The listing builds one solid part. Answer for the finished solid, in the listing's coordinates (mm). A direction names the side the tool comes from. Give positions to 0.01 mm unless a question says otherwise; leave off trailing zeros. Loops run counter-clockwise (first coordinate to the right, second up) from the corner with the lowest first, then second, coordinate; pieces in that order, holes last. Notation, with made-up numbers: M 86.25,72.5 L 127.25,72.5 A9 cw 127.25,82.5 Z; hole C 60,22.25 d7. An arc over 180 degrees is marked long. Use one line per item in the form item = value. Start each with the question number.
1. The part is cut by section D-D (x = 43). Write down the section's boundary in (y, z), and give its area (3 significant figures).
2. The part is cut by section A-A (z = 66.5). Write down the section's boundary in (x, y), and give its area (3 significant figures).
3. The part is cut by section C-C (z = 20). Give the number of separate pieces and of enclosed holes in the cut face, and give its area (3 significant figures).
4. Straight lines are drawn through the part: line 1 (X direction, y = -25.5, z = 46); line 2 (X direction, y = -80.5, z = 25); line 3 (Z direction, x = -117, y = 64). For each, find the intervals that lie inside material, in ascending order. Write a range as from..to.
5. The mould has two halves that part along X. Classify faces 5 (the face through (-118, -107.883, 26)), 6 (the face through (141.234, 24, 40)), 7 (the face through (125, -107.883, 26)), 8 (the face through (130, -24.883, 30)): released by +X, released by -X, zero draft, split by the parting line, or undercut.
6. For faces 1 (the face through (127, -19.883, 27)), 2 (the face through (-118, 65.117, 26)), 3 (the face through (-133.766, 24, 40)), 4 (the face through (24.2, -112.883, 4.5)), determine the directions among +Z, -Z, +X, -X, +Y, -Y from which every point of the face is accessible in a straight line to the end or side of a thin tool.
7. The part is cut by section B-B (y = 20). Write down the section's boundary in (x, z).
8. Each of these flat-tipped pins is pushed along its axis until it touches: pin 1 Ø1 at (y, z) = (-47, 14) entering from -X; pin 2 Ø24 at (y, z) = (-57, 29) entering from +X; pin 3 Ø13.5 at (x, z) = (128, 40.5) entering from +Y. Where does it stop, or does it pass through?
from build123d import *

# Parameters (mm, degrees)
SKETCH1_W                = 285
SKETCH1_H                = 188
BOSS_EXTRUDE1_DEPTH      = 5
SKETCH3_W                = 5
SKETCH3_H                = 90
BOSS_EXTRUDE2_DEPTH      = 72
SKETCH6_W                = 40
SKETCH6_H                = 5
BOSS_EXTRUDE3_DEPTH      = 10
SKETCH7_W                = 12
SKETCH7_H                = 5
BOSS_EXTRUDE4_DEPTH      = 45
SKETCH8_W                = 40
SKETCH8_H                = 5
BOSS_EXTRUDE5_DEPTH      = 72
CUT_EXTRUDE4_DEPTH       = 94
CUT_EXTRUDE4_DEPTH_BACK  = 96
SKETCH13_W               = 5
SKETCH13_H               = 90
BOSS_EXTRUDE6_DEPTH      = 72
SKETCH14_W               = 40
SKETCH14_H               = 5
BOSS_EXTRUDE7_DEPTH      = 55
SKETCH16_W               = 28
SKETCH16_H               = 45
CUT_EXTRUDE5_DEPTH       = 179
CUT_EXTRUDE5_DEPTH_BACK  = 11
SKETCH17_W               = 40
SKETCH17_H               = 5
BOSS_EXTRUDE9_DEPTH      = 55
SKETCH21_W               = 27.761976985
SKETCH21_H               = 40
CUT_EXTRUDE6_DEPTH       = 91
CUT_EXTRUDE6_DEPTH_BACK  = 99
SKETCH22_W               = 5
SKETCH22_H               = 88
BOSS_EXTRUDE10_DEPTH     = 80
SKETCH23_W               = 40
SKETCH23_H               = 5
BOSS_EXTRUDE11_DEPTH     = 55
SKETCH25_W               = 27.891782469
SKETCH25_H               = 44.37316573
CUT_EXTRUDE7_DEPTH       = 184
CUT_EXTRUDE7_DEPTH_BACK  = 6
SKETCH26_W               = 40
SKETCH26_H               = 5
BOSS_EXTRUDE12_DEPTH     = 55
SKETCH27_W               = 28
SKETCH27_H               = 45
CUT_EXTRUDE9_DEPTH       = 101
CUT_EXTRUDE9_DEPTH_BACK  = 89
SKETCH29_W               = 5
SKETCH29_H               = 88
BOSS_EXTRUDE14_DEPTH     = 80
SKETCH30_W               = 40
SKETCH30_H               = 5
BOSS_EXTRUDE15_DEPTH     = 55
SKETCH31_W               = 27.846515173
SKETCH31_H               = 45
CUT_EXTRUDE10_DEPTH      = 184
CUT_EXTRUDE10_DEPTH_BACK = 6
SKETCH32_W               = 40
SKETCH32_H               = 5
BOSS_EXTRUDE16_DEPTH     = 55
SKETCH33_W               = 27.846515173
SKETCH33_H               = 45
CUT_EXTRUDE11_DEPTH      = 84
CUT_EXTRUDE11_DEPTH_BACK = 106
SKETCH36_W               = 15
SKETCH36_H               = 5
CUT_EXTRUDE12_DEPTH      = 1
CUT_EXTRUDE12_DEPTH_BACK = 7


with BuildPart() as part:
    # Sketch1 → Boss-Extrude1 (new body)
    with BuildSketch(Plane.XY):
        with Locations((3.734064661, -18.883040936)):
            Rectangle(SKETCH1_W, SKETCH1_H)
    extrude(amount=BOSS_EXTRUDE1_DEPTH)

    # Sketch3 → Boss-Extrude2 (add)
    with BuildSketch(Plane.XY.offset(5)):
        with Locations((-131.265935339, 25.116959064)):
            Rectangle(SKETCH3_W, SKETCH3_H)
    extrude(amount=BOSS_EXTRUDE2_DEPTH)

    # Sketch6 → Boss-Extrude3 (add)
    with BuildSketch(Plane.XY.offset(5)):
        with Locations((-108.765935339, 67.616959064)):
            Rectangle(SKETCH6_W, SKETCH6_H)
    extrude(amount=BOSS_EXTRUDE3_DEPTH)

    # Sketch7 → Boss-Extrude4 (add)
    with BuildSketch(Plane.XY.offset(15)):
        with Locations((-122.765935339, 67.616959064)):
            Rectangle(SKETCH7_W, SKETCH7_H)
    extrude(amount=BOSS_EXTRUDE4_DEPTH)

    # Sketch8 → Boss-Extrude5 (add)
    with BuildSketch(Plane.XY.offset(77)):
        with Locations((-108.765935339, -17.383040936)):
            Rectangle(SKETCH8_W, SKETCH8_H)
    extrude(amount=-BOSS_EXTRUDE5_DEPTH)

    # Sketch9 → Cut-Extrude4 (cut, two sides)
    with BuildSketch(Plane.XZ.offset(19.883040936)) as cut_extrude4_sk:
        Polygon((-116.765935339, 15), (-88.765935339, 15), (-88.765935339, 77), (-128.765935339, 77), (-128.765935339, 60), (-116.765935339, 60), align=None)
    extrude(amount=CUT_EXTRUDE4_DEPTH, mode=Mode.SUBTRACT)
    extrude(cut_extrude4_sk.sketch, amount=-CUT_EXTRUDE4_DEPTH_BACK, mode=Mode.SUBTRACT)

    # Sketch13 → Boss-Extrude6 (add)
    with BuildSketch(Plane.XY.offset(5)):
        with Locations((138.734064661, 25.116959064)):
            Rectangle(SKETCH13_W, SKETCH13_H)
    extrude(amount=BOSS_EXTRUDE6_DEPTH)

    # Sketch14 → Boss-Extrude7 (add)
    with BuildSketch(Plane.XY.offset(5)):
        with Locations((116.234064661, 67.616959064)):
            Rectangle(SKETCH14_W, SKETCH14_H)
    extrude(amount=BOSS_EXTRUDE7_DEPTH)

    # Sketch16 → Cut-Extrude5 (cut, two sides)
    with BuildSketch(Plane.XZ.offset(-65.116959064)) as cut_extrude5_sk:
        with Locations((110.234064661, 37.5)):
            Rectangle(SKETCH16_W, SKETCH16_H)
    extrude(amount=CUT_EXTRUDE5_DEPTH, mode=Mode.SUBTRACT)
    extrude(cut_extrude5_sk.sketch, amount=-CUT_EXTRUDE5_DEPTH_BACK, mode=Mode.SUBTRACT)

    # Sketch17 → Boss-Extrude9 (add)
    with BuildSketch(Plane.XY):
        with Locations((116.234064661, -17.383040936)):
            Rectangle(SKETCH17_W, SKETCH17_H)
    extrude(amount=BOSS_EXTRUDE9_DEPTH)

    # Sketch21 → Cut-Extrude6 (cut, two sides)
    with BuildSketch(Plane(origin=(0, -14.883040936, 0), x_dir=(1, 0, 0), z_dir=(0, 1, 0))) as cut_extrude6_sk:
        with Locations((110.115053154, -35)):
            Rectangle(SKETCH21_W, SKETCH21_H)
    extrude(amount=CUT_EXTRUDE6_DEPTH, mode=Mode.SUBTRACT)
    extrude(cut_extrude6_sk.sketch, amount=-CUT_EXTRUDE6_DEPTH_BACK, mode=Mode.SUBTRACT)

    # Sketch22 → Boss-Extrude10 (add)
    with BuildSketch(Plane.XY.offset(5)):
        with Locations((-131.265935339, -68.883040936)):
            Rectangle(SKETCH22_W, SKETCH22_H)
    extrude(amount=BOSS_EXTRUDE10_DEPTH)

    # Sketch23 → Boss-Extrude11 (add)
    with BuildSketch(Plane.XY.offset(5)):
        with Locations((-108.765935339, -110.383040936)):
            Rectangle(SKETCH23_W, SKETCH23_H)
    extrude(amount=BOSS_EXTRUDE11_DEPTH)

    # Sketch25 → Cut-Extrude7 (cut, two sides)
    with BuildSketch(Plane(origin=(0, -107.883040936, 0), x_dir=(1, 0, 0), z_dir=(0, 1, 0))) as cut_extrude7_sk:
        with Locations((-102.711826574, -37.813417135)):
            Rectangle(SKETCH25_W, SKETCH25_H)
    extrude(amount=CUT_EXTRUDE7_DEPTH, mode=Mode.SUBTRACT)
    extrude(cut_extrude7_sk.sketch, amount=-CUT_EXTRUDE7_DEPTH_BACK, mode=Mode.SUBTRACT)

    # Sketch26 → Boss-Extrude12 (add)
    with BuildSketch(Plane.XY.offset(5)):
        with Locations((-108.765935339, -27.383040936)):
            Rectangle(SKETCH26_W, SKETCH26_H)
    extrude(amount=BOSS_EXTRUDE12_DEPTH)

    # Sketch27 → Cut-Extrude9 (cut, two sides)
    with BuildSketch(Plane(origin=(0, -24.883040936, 0), x_dir=(1, 0, 0), z_dir=(0, 1, 0))) as cut_extrude9_sk:
        with Locations((-102.765935339, -37.5)):
            Rectangle(SKETCH27_W, SKETCH27_H)
    extrude(amount=CUT_EXTRUDE9_DEPTH, mode=Mode.SUBTRACT)
    extrude(cut_extrude9_sk.sketch, amount=-CUT_EXTRUDE9_DEPTH_BACK, mode=Mode.SUBTRACT)

    # Sketch29 → Boss-Extrude14 (add)
    with BuildSketch(Plane.XY.offset(5)):
        with Locations((138.734064661, -68.883040936)):
            Rectangle(SKETCH29_W, SKETCH29_H)
    extrude(amount=BOSS_EXTRUDE14_DEPTH)

    # Sketch30 → Boss-Extrude15 (add)
    with BuildSketch(Plane.XY.offset(5)):
        with Locations((116.234064661, -110.383040936)):
            Rectangle(SKETCH30_W, SKETCH30_H)
    extrude(amount=BOSS_EXTRUDE15_DEPTH)

    # Sketch31 → Cut-Extrude10 (cut, two sides)
    with BuildSketch(Plane(origin=(0, -107.883040936, 0), x_dir=(1, 0, 0), z_dir=(0, 1, 0))) as cut_extrude10_sk:
        with Locations((110.157322248, -37.5)):
            Rectangle(SKETCH31_W, SKETCH31_H)
    extrude(amount=CUT_EXTRUDE10_DEPTH, mode=Mode.SUBTRACT)
    extrude(cut_extrude10_sk.sketch, amount=-CUT_EXTRUDE10_DEPTH_BACK, mode=Mode.SUBTRACT)

    # Sketch32 → Boss-Extrude16 (add)
    with BuildSketch(Plane.XY.offset(5)):
        with Locations((116.234064661, -27.383040936)):
            Rectangle(SKETCH32_W, SKETCH32_H)
    extrude(amount=BOSS_EXTRUDE16_DEPTH)

    # Sketch33 → Cut-Extrude11 (cut, two sides)
    with BuildSketch(Plane.XZ.offset(29.883040936)) as cut_extrude11_sk:
        with Locations((110.157322248, 37.5)):
            Rectangle(SKETCH33_W, SKETCH33_H)
    extrude(amount=CUT_EXTRUDE11_DEPTH, mode=Mode.SUBTRACT)
    extrude(cut_extrude11_sk.sketch, amount=-CUT_EXTRUDE11_DEPTH_BACK, mode=Mode.SUBTRACT)

    # Sketch36 → Cut-Extrude12 (cut, two sides)
    with BuildSketch(Plane(origin=(0, 75.116959064, 0), x_dir=(1, 0, 0), z_dir=(0, 1, 0))) as cut_extrude12_sk:
        with Locations((3.734064661, -2.5)):
            Rectangle(SKETCH36_W, SKETCH36_H)
    extrude(amount=CUT_EXTRUDE12_DEPTH, mode=Mode.SUBTRACT)
    extrude(cut_extrude12_sk.sketch, amount=-CUT_EXTRUDE12_DEPTH_BACK, mode=Mode.SUBTRACT)


solid = part.part
Derived:
q1.outline = M -112.88,0 L 75.12,0 L 75.12,5 L -112.88,5 Z
q1.area = 940 mm2
q2.outline = M -133.77,-112.88 L -128.77,-112.88 L -128.77,-24.88 L -133.77,-24.88 Z; M -133.77,-19.88 L -128.77,-19.88 L -128.77,70.12 L -133.77,70.12 Z; M 136.23,-112.88 L 141.23,-112.88 L 141.23,-24.88 L 136.23,-24.88 Z; M 136.23,-19.88 L 141.23,-19.88 L 141.23,70.12 L 136.23,70.12 Z
q2.area = 1,780 mm2
q3.separate_pieces = 4
q3.enclosed_holes = 0
q3.area = 2,260 mm2
q4.line_1 = -133.77..-116.77, 124.08..141.23
q4.line_2 = -133.77..-128.77, 136.23..141.23
q4.line_3 = 0..5
q5.face_5 = undercut
q5.face_6 = released by +X
q5.face_7 = undercut
q5.face_8 = zero draft
q6.face_1 = +Z, +X, -X
q6.face_2 = +Z
q6.face_3 = +Z, -X, +Y, -Y
q6.face_4 = +Z, -Z, +X, -X, -Y
q7.outline = M -138.77,0 L 146.23,0 L 146.23,5 L 141.23,5 L 141.23,77 L 136.23,77 L 136.23,5 L -128.77,5 L -128.77,77 L -133.77,77 L -133.77,5 L -138.77,5 Z
q8.pin_1 = -133.77
q8.pin_2 = 141.23
q8.pin_3 = 70.12
